Geometry check sheet. Reference: the model listing, model coordinates, mm. A direction names the side the tool comes from. Give positions to 0.01 mm unless a question says otherwise; leave off trailing zeros. Write each loop counter-clockwise with the first axis right and the second up, starting at its lowest first coordinate (ties: lowest second). Pieces come first, ordered by that corner, then holes. Notation, with made-up numbers: (-27, 36.5) - (-12, 36.5) arc R14 cw to (-12, 57.5) - close; hole circle Ø4 at (57, 31.5). An arc over 180 degrees is marked (long way). Write item = value, one per line. Start each with the question number.
(1) Section check A-A, the plane z = -55. Enter the section's corners in (x, y), plus the area to 3 significant figures.
(2) Section check C-C, the plane x = 26.5. Enter the section's corners in (y, z), plus the area to 3 significant figures.
(3) Section check B-B, the plane y = 494.5. Enter the section's corners in (x, z), plus the area to 3 significant figures.
(4) Draft check along X on faces 1 (the flat face through (8, 246, -45)), 2 (the flat face through (10.753, 557.685, -3.944)), 3 (the flat face through (75, 500, -41)). Enter one of: pulls with the +X half, pulls with the -X half, needs draft (parallel to the pull), parting line crosses it, or undercut.
(5) Depth check by flat-ended pin: pin 1 Ø5 at (x, y) = (58.5, 526.5) entering from -Z; pin 2 Ø1.2 at (y, z) = (501, -5) entering from -X; pin 3 Ø4 at (x, z) = (5, -37.5) entering from +Y. Enter the tip coordinate at first touch or a pass-through.
(6) Access from +Z, -Z, +X, -X, +Y, -Y to the whole of each face (thin tool, end or side, straight path). Record for faces 4 (the flat face through (39, 305, 0)), 5 (the flat face through (5, 500, -41)), 6 (the flat face through (72, 254, -45)).
(7) Thickness scan on L1, parallel to X at y = 416, z = -8.5; L2, parallel to Y at x = 74, z = -41.5; L3, parallel to Z at x = 61, y = 494.5. Record the ranges inside material, lowest first.
```python
from build123d import *

# Parameters (mm, degrees)
SKETCH_1_R                        = 5
SM_BASE_FLANGE_2_DEPTH            = 8
SM_EDGE_FLANGE_4_STRIP_W          = 33.4732
SM_EDGE_FLANGE_4_STRIP_H          = 8
SM_EDGE_FLANGE_4_STRIP_CUT_DEPTH  = 500
SM_EDGE_FLANGE_4_RELIEF_W         = 37.4732
SM_EDGE_FLANGE_4_RELIEF_H         = 4
SM_EDGE_FLANGE_4_RELIEF_CUT_DEPTH = 8
SM_EDGE_FLANGE_4_DEPTH            = 500
SM_EDGE_FLANGE_8_STRIP_W          = 33.4732
SM_EDGE_FLANGE_8_STRIP_H          = 8
SM_EDGE_FLANGE_8_STRIP_CUT_DEPTH  = 500
SM_EDGE_FLANGE_8_RELIEF_W         = 37.4732
SM_EDGE_FLANGE_8_RELIEF_H         = 4
SM_EDGE_FLANGE_8_RELIEF_CUT_DEPTH = 8
SM_EDGE_FLANGE_8_DEPTH            = 500


# Sheet-metal steps are written as plain solids
with BuildPart() as part:
    # 草图1 → 基体-法兰2 (new body)
    with BuildSketch(Plane.XY):
        with BuildLine():
            Line((0, 0), (80, 0))
            Line((80, 0), (80, 520))
            Line((80, 520), (58.758007847, 594.277403974))
            ThreePointArc((58.758007847, 594.277403974), (39.983985428, 600.877915043), (21.209963009, 594.277403974))
            Line((21.209963009, 594.277403974), (0, 520.054307268))
            Line((0, 520.054307268), (0, 0))
        make_face()
        with Locations((39.983985428, 570.877915043)):
            Circle(SKETCH_1_R, mode=Mode.SUBTRACT)
        with Locations((39.983985428, 550.877915043)):
            Circle(SKETCH_1_R, mode=Mode.SUBTRACT)
        with Locations((39.983985428, 530.877915043)):
            Circle(SKETCH_1_R, mode=Mode.SUBTRACT)
    extrude(amount=-SM_BASE_FLANGE_2_DEPTH)

    # 边线-法兰4 strip (across the edge) → 边线-法兰4 strip cut (cut)
    with BuildSketch(Plane(origin=(0, 0, -8), x_dir=(1, 0, 0), z_dir=(0, 1, 0))):
        with Locations((-8, -4)):
            Rectangle(SM_EDGE_FLANGE_4_STRIP_W, SM_EDGE_FLANGE_4_STRIP_H)
    extrude(amount=SM_EDGE_FLANGE_4_STRIP_CUT_DEPTH, mode=Mode.SUBTRACT)

    # 边线-法兰4 relief (on the sheet) → 边线-法兰4 relief cut (cut)
    with BuildSketch(Plane(origin=(8.7366, 0, -8), x_dir=(1, 0, 0), z_dir=(0, 0, -1))):
        with Locations((-14.7366, -502)):
            Rectangle(SM_EDGE_FLANGE_4_RELIEF_W, SM_EDGE_FLANGE_4_RELIEF_H)
    extrude(amount=-SM_EDGE_FLANGE_4_RELIEF_CUT_DEPTH, mode=Mode.SUBTRACT)

    # 边线-法兰4 section (across the edge) → 边线-法兰4 (add)
    with BuildSketch(Plane(origin=(0, 0, -8), x_dir=(1, 0, 0), z_dir=(0, 1, 0))):
        with BuildLine():
            Line((0, 0.7366), (0, 72))
            Line((0, 72), (8, 72))
            Line((8, 72), (8, 0.7366))
            ThreePointArc((8, 0.7366), (8.215745145, 0.215745145), (8.7366, 0))
            Line((8.7366, 0), (8.7366, -8))
            ThreePointArc((8.7366, -8), (2.558890895, -5.441109105), (0, 0.7366))
        make_face()
    extrude(amount=SM_EDGE_FLANGE_4_DEPTH)

    # 边线-法兰8 strip (across the edge) → 边线-法兰8 strip cut (cut)
    with BuildSketch(Plane(origin=(80, 500, -8), x_dir=(-1, 0, 0), z_dir=(0, -1, 0))):
        with Locations((-8, -4)):
            Rectangle(SM_EDGE_FLANGE_8_STRIP_W, SM_EDGE_FLANGE_8_STRIP_H)
    extrude(amount=SM_EDGE_FLANGE_8_STRIP_CUT_DEPTH, mode=Mode.SUBTRACT)

    # 边线-法兰8 relief (on the sheet) → 边线-法兰8 relief cut (cut)
    with BuildSketch(Plane(origin=(71.2634, 500, -8), x_dir=(-1, 0, 0), z_dir=(0, 0, -1))):
        with Locations((-14.7366, 2)):
            Rectangle(SM_EDGE_FLANGE_8_RELIEF_W, SM_EDGE_FLANGE_8_RELIEF_H)
    extrude(amount=-SM_EDGE_FLANGE_8_RELIEF_CUT_DEPTH, mode=Mode.SUBTRACT)

    # 边线-法兰8 section (across the edge) → 边线-法兰8 (add)
    with BuildSketch(Plane(origin=(80, 500, -8), x_dir=(-1, 0, 0), z_dir=(0, -1, 0))):
        with BuildLine():
            Line((0, 0.7366), (0, 72))
            Line((0, 72), (8, 72))
            Line((8, 72), (8, 0.7366))
            ThreePointArc((8, 0.7366), (8.215745145, 0.215745145), (8.7366, 0))
            Line((8.7366, 0), (8.7366, -8))
            ThreePointArc((8.7366, -8), (2.558890895, -5.441109105), (0, 0.7366))
        make_face()
    extrude(amount=SM_EDGE_FLANGE_8_DEPTH)


solid = part.part
```
Model answer:
q1.outline = (0, 0) - (8, 0) - (8, 500) - (0, 500) - close; (72, 0) - (80, 0) - (80, 500) - (72, 500) - close
q1.area = 8,000 mm²
q2.outline = (0, -8) - (597.68, -8) - (597.68, 0) - (0, 0) - close
q2.area = 4,780 mm²
q3.outline = (0, -80) - (8, -80) - (8, -8.74) arc R0.74 cw to (8.74, -8) - (71.26, -8) arc R0.74 cw to (72, -8.74) - (72, -80) - (80, -80) - (80, -8.74) arc R8.74 ccw to (71.26, 0) - (8.74, 0) arc R8.74 ccw to (0, -8.74) - close
q3.area = 1,760 mm²
q4.face_1 = undercut
q4.face_2 = pulls with the -X half
q4.face_3 = needs draft
q5.pin_1 = -8
q5.pin_2 = 12.74
q5.pin_3 = 500
q6.face_4 = +Z, +X, -X, +Y, -Y
q6.face_5 = +Z, -Z, -X
q6.face_6 = -Z, +Y, -Y
q7.L1 = 0 to 8.04, 71.96 to 80
q7.L2 = 0 to 500
q7.L3 = -8 to 0
